```python
from build123d import *

# Parameters (mm, degrees)
SKETCH1_R           = 1.25
BOSS_EXTRUDE1_DEPTH = 2.4
SKETCH2_R           = 2.75
SKETCH2_R_2         = 1.25
BOSS_EXTRUDE2_DEPTH = 1.6
FILLET1_R           = 0.2
FILLET2_R           = 0.8


with BuildPart() as part:
    # Sketch1 → Boss-Extrude1 (new body)
    with BuildSketch(Plane.XY):
        Polygon((3.175426481, 0), (1.58771324, 2.75), (-1.58771324, 2.75), (-3.175426481, 0), (-1.58771324, -2.75), (1.58771324, -2.75), align=None)
        Circle(SKETCH1_R, mode=Mode.SUBTRACT)
    extrude(amount=BOSS_EXTRUDE1_DEPTH)

    # Sketch2 → Boss-Extrude2 (add)
    with BuildSketch(Plane.XY.offset(2.4)):
        Circle(SKETCH2_R)
        Circle(SKETCH2_R_2, mode=Mode.SUBTRACT)
    extrude(amount=BOSS_EXTRUDE2_DEPTH)

    # Fillet1
    fillet1_edges = [part.edges().sort_by_distance(p)[0] for p in [
        (-1.25, 0, 0),
        (0, -2.75, 0),
        (-2.38156986, -1.375, 0),
        (-2.38156986, 1.375, 0),
        (0, 2.75, 0),
        (2.38156986, 1.375, 0),
        (2.38156986, -1.375, 0),
    ]]
    fillet(fillet1_edges, radius=FILLET1_R)

    # Fillet2
    fillet2_edges = [part.edges().sort_by_distance(p)[0] for p in [
        (-2.75, 0, 4),
    ]]
    fillet(fillet2_edges, radius=FILLET2_R)


solid = part.part
```
CAD build for the part. Positions are in the model's coordinates, mm. A direction names the side the tool comes from. Round coordinates to 2 decimals unless told otherwise and drop trailing zeros. Write each loop counter-clockwise with the first axis right and the second up, starting at its lowest first coordinate (ties: lowest second). Pieces come first, ordered by that corner, then holes. Notation, with made-up numbers: (80.5, 2.5) - (132.5, 2.5) arc R22 ccw to (132.5, 8.5) - close; hole circle Ø4 at (54, -2.5). An arc over 180 degrees is marked (long way). Return JSON: item names as keys, results as strings. Group by question number.
Item 1: Band-saw the part on A-A on z = 2.1. List the corners of the cut face in (x, y).
Item 2: Probe probe 1 along Y at (x, z) = (0, 1.7); probe 2 along X at (y, z) = (-0.95, 0.4); probe 3 along X at (y, z) = (-1, 2.2). List the from-to ranges inside material, lowest first.
Item 3: 3-axis set-ups, long thin cutter, end or side, ignore diameter. For faces 4 (the face through (-0.596, -2.685, 2.794)), 5 (the face through (-1.5, 2.5, 2.4)), 6 (the face through (-1.5, -2.5, 2.4)): which of +Z, -Z, +X, -X, +Y, -Y reach the whole face in a straight line?
Item 4: Flat gauge pins, fed straight in: pin 1 Ø1.1 at (x, y) = (1.5, -2) entering from +Z; pin 2 Ø0.9 at (x, y) = (3, 0.5) entering from +Z; pin 3 Ø2 at (x, y) = (0, 0) entering from -Z. Where does each tip first touch, or does it go through?
Item 5: Band-saw the part on B-B on z = 2.7. List the corners of the cut face in (x, y), plus the area to 3 significant figures.
Item 6: Mould opens along X. For faces 1 (the face through (-2.39, -1.36, 1.28)), 2 (the face through (-0.27, -1.22, 2.07)), 3 (the face through (0, -2.75, 1)) say: +X half, -X half, draft (parallel to the pull), parting line (faces both ways), or undercut.
Resolved:
{
 "1": {"outline": "(-3.18, 0) - (-1.59, -2.75) - (1.59, -2.75) - (3.18, 0) - (1.59, 2.75) - (-1.59, 2.75) - close; hole circle Ø2.5 at (0, 0)"},
 "2": {"probe 1": "y = -2.75 to -1.25, 1.25 to 2.75", "probe 2": "x = -2.63 to -0.81, 0.81 to 2.63", "probe 3": "x = -2.6 to -0.75, 0.75 to 2.6"},
 "3": {"face 4": "+Z", "face 5": "+Z, -X, +Y", "face 6": "+Z, -X, -Y"},
 "4": {"pin 1": "stops at z = 4", "pin 2": "stops at z = 3.68", "pin 3": "passes through"},
 "5": {"outline": "circle Ø5.5 at (0, 0); hole circle Ø2.5 at (0, 0)", "area": "18.8 mm²"},
 "6": {"face 1": "-X half", "face 2": "undercut", "face 3": "draft"}
}
